Answer from the drawing. Dimensions are ordinates in mm from the lowest x, y and z of the part. A direction names the side the tool comes from. Round coordinates to 2 decimals unless told otherwise and drop trailing zeros. Order: outer loops, then holes, each group sorted by start corner. A loop starts at its lowest first (then second) coordinate and runs counter-clockwise, first axis right, second up. Notation, with made-up numbers: (-32.75, 76.25) - (-24.75, 76.25) arc R12 cw to (-24.75, 87.25) - close; hole circle Ø5 at (49, 20). An arc over 180 degrees is marked (long way). One line per question, with ' | ' between items. Start each with the question number.
1) The part is cut by section D-D, the plane z = 1.2. Count the separate pieces of the cut face and the enclosed holes in it, plus the area to 3 significant figures.
2) Straight lines are drawn through the part: line 1 (Y direction, x = 10, z = 2.8); line 2 (Y direction, x = 9.25, z = 3.45); line 3 (Z direction, x = 6, y = 3.5). For each, find the intervals that lie inside material, in ascending order. Write a range as from..to.
3) For the marked faces 4 and 5, determine the directions among +Z, -Z, +X, -X, +Y, -Y from which every point of the face is accessible in a straight line to the end or side of a thin tool.
4) The part is cut by section A-A, the plane y = 10. Give the vertices of the cut face in (x, z).
5) The mould has two halves that part along Y. Classify the marked faces 1, 2 and 3: pulls with the +Y half, pulls with the -Y half, needs draft (parallel to the pull), parting line crosses it, or undercut.
6) Flat-ended cylindrical pins translate along their axes: pin 1 (1.6 mm diameter, centred on x = 14.95, y = 14.95, fed in from +Z); pin 2 (1.5 mm diameter, centred on x = 12, y = 2.5, fed in from +Z); pin 3 (1.5 mm diameter, centred on x = 5.5, y = 8.5, fed in from -Z); pin 4 (1.5 mm diameter, centred on x = 5, z = 4, fed in from +Y). Find the tip coordinate at first contact, or state that the pin passes through.
7) The part is cut by section B-B, the plane x = 17. Give the vertices of the cut face in (y, z).
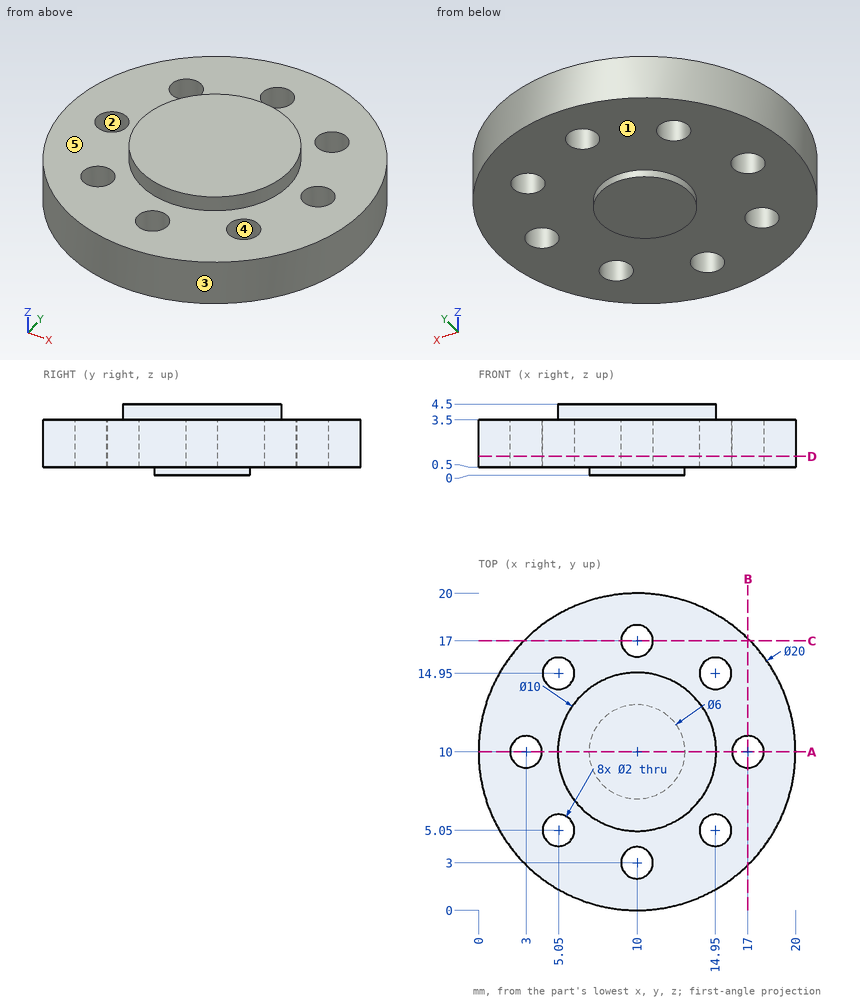
Values:
1) separate pieces: 1 | enclosed holes: 8 | area: 289 mm^2
2) line 1: y = 0..2, 4..16, 18..20 | line 2: y = 0.03..2.34, 3.66..16.34, 17.66..19.97 | line 3: z = 0.5..3.5
3) face 4: +Z, -Z | face 5: +Z
4) outline: (0, 0.5) - (2, 0.5) - (2, 3.5) - (0, 3.5) - close; (4, 0.5) - (7, 0.5) - (7, 0) - (13, 0) - (13, 0.5) - (16, 0.5) - (16, 3.5) - (15, 3.5) - (15, 4.5) - (5, 4.5) - (5, 3.5) - (4, 3.5) - close; (18, 0.5) - (20, 0.5) - (20, 3.5) - (18, 3.5) - close
5) face 1: needs draft | face 2: undercut | face 3: parting line crosses it
6) pin 1: passes through | pin 2: stops at z = 3.5 | pin 3: stops at z = 0.5 | pin 4: stops at y = 18.96
7) outline: (2.86, 0.5) - (9, 0.5) - (9, 3.5) - (2.86, 3.5) - close; (11, 0.5) - (17.14, 0.5) - (17.14, 3.5) - (11, 3.5) - close
